Geometry: see drawing. Coordinates: mm, zero at the bounding-box minimum. A direction names the side the tool comes from. Coordinates: 2 decimals unless noted, no trailing zeros. Write each loop counter-clockwise with the first axis right and the second up, starting at its lowest first coordinate (ties: lowest second). Pieces come first, ordered by that corner, then holes. Notation, with made-up numbers: (71.5, 72.5) - (116.5, 72.5) arc R16 ccw to (116.5, 82.5) - close; hole circle Ø9 at (53.25, -1). An arc over 180 degrees is marked (long way). Use a Markdown table: item, result. Add a question column.
Q1. Material intervals for probe 1 along Z at (x, y) = (7, 7); probe 2 along X at (y, z) = (8, 5); probe 3 along Z at (x, y) = (5.25, 12.75), sorted ascending. Write a range as from..to.
Q2. Section query C-C (z = 6.5). Return the cut outline in (x, y).
Q3. Mould query, pull axis Z, two halves, no side actions, for the marked faces 4, 5 and 6. Classes: released by +Z, released by -Z, zero draft, split by the parting line, or undercut.
Q4. Section query D-D (z = 9.5). Return the cut outline in (x, y) (1 decimal).
Q5. Section query A-A (y = 13.25). Return the cut outline in (x, z).
Q6. Section query B-B (x = 6.25). Return the cut outline in (y, z).
Q7. Pin query (flat end, axial travel): P1, Ø1, axis at x = 7, z = 10.5, coming from the -Y side; P2, Ø3, axis at y = 3, z = 9, coming from the -X side; P3, Ø6, axis at x = 2, y = 3.5, coming from the +Z side. Return the tip coordinate at first contact, or that it passes through.
Q8. Set-up query: the marked faces 1, 2 and 3. Return all of +Z, -Z, +X, -X, +Y, -Y with unobstructed straight access to the full face (end or side cutting, diameter ignored); none if empty.
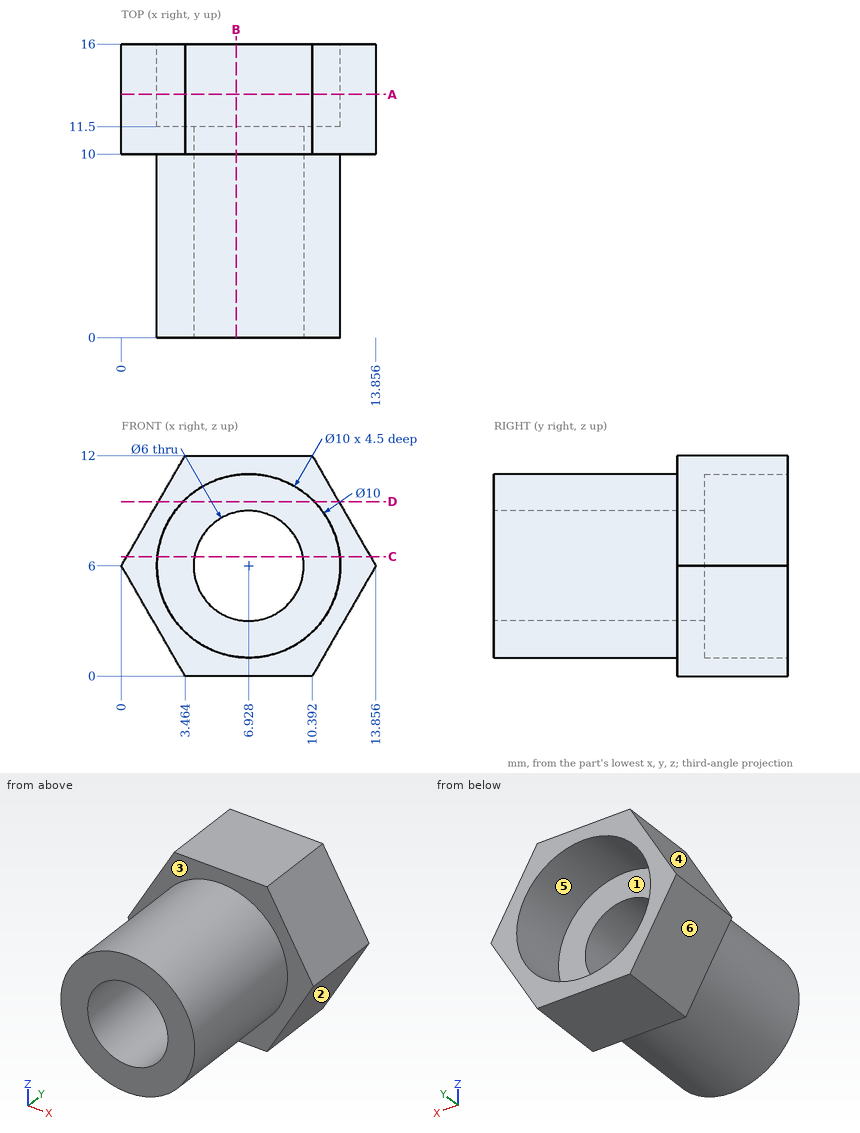
Values follow:
| question | item | result |
|---|---|---|
| 1 | probe 1 | 1..3, 9..11 |
| 1 | probe 2 | 2.03..4.1, 9.76..11.83 |
| 1 | probe 3 | 0..1.29, 10.71..12 |
| 2 | outline | (0.29, 10) - (1.95, 10) - (1.95, 0) - (3.97, 0) - (3.97, 11.5) - (1.95, 11.5) - (1.95, 16) - (0.29, 16) - close; (9.89, 0) - (11.9, 0) - (11.9, 10) - (13.57, 10) - (13.57, 16) - (11.9, 16) - (11.9, 11.5) - (9.89, 11.5) - close |
| 3 | face 4 | released by +Z |
| 3 | face 5 | undercut |
| 3 | face 6 | released by -Z |
| 4 | outline | (2, 10) - (3.4, 10) - (3.4, 0) - (10.5, 0) - (10.5, 10) - (11.8, 10) - (11.8, 16) - (10.5, 16) - (10.5, 11.5) - (3.4, 11.5) - (3.4, 16) - (2, 16) - close |
| 5 | outline | (0, 6) - (3.46, 0) - (10.39, 0) - (13.86, 6) - (10.39, 12) - (3.46, 12) - close; hole circle Ø10 at (6.93, 6) |
| 6 | outline | (0, 1.05) - (10, 1.05) - (10, 0) - (16, 0) - (16, 1.05) - (11.5, 1.05) - (11.5, 3.08) - (0, 3.08) - close; (0, 8.92) - (11.5, 8.92) - (11.5, 10.95) - (16, 10.95) - (16, 12) - (10, 12) - (10, 10.95) - (0, 10.95) - close |
| 7 | P1 | y = 0 |
| 7 | P2 | x = 2.16 |
| 7 | P3 | z = 10.61 |
| 8 | face 1 | +Y |
| 8 | face 2 | -Z, +X, +Y, -Y |
| 8 | face 3 | -Y |
